```python
from build123d import *

# Parameters (mm, degrees)
SZKIC1_R                    = 3
DODANIE_WYCI_GNI_CIE1_DEPTH = 30
DODANIE_WYCI_GNI_CIE2_DEPTH = 4
SFAZOWANIE1_SIZE            = 1


with BuildPart() as part:
    # Szkic1 → Dodanie-wyciągnięcie1 (new body)
    with BuildSketch(Plane(origin=(0, 0, 0), x_dir=(1, 0, 0), z_dir=(0, 1, 0))):
        with Locations(Location((0, 0, 0), (0, 0, 270))):
            Circle(SZKIC1_R)
    extrude(amount=-DODANIE_WYCI_GNI_CIE1_DEPTH)

    # Szkic2 → Dodanie-wyciągnięcie2 (add)
    with BuildSketch(Plane(origin=(0, 0, 0), x_dir=(1, 0, 0), z_dir=(0, 1, 0))):
        Polygon((5.773502692, 0), (2.886751346, 5), (-2.886751346, 5), (-5.773502692, 0), (-2.886751346, -5), (2.886751346, -5), align=None)
    extrude(amount=DODANIE_WYCI_GNI_CIE2_DEPTH)

    # Szkic4 → Wycięcie-obrót1 (revolve, cut)
    with BuildSketch(Plane.XY):
        Polygon((5.773502692, 3.226497308), (5, 4), (5.773502692, 4), align=None)
    revolve(axis=Axis((0, 4, 0), (0, -1, 0)), mode=Mode.SUBTRACT)

    # Sfazowanie1
    sfazowanie1_edges = [part.edges().sort_by_distance(p)[0] for p in [
        (0, -30, -3),
    ]]
    chamfer(sfazowanie1_edges, length=SFAZOWANIE1_SIZE)


solid = part.part
```
Model file for the job. Use its own axes, mm. A direction names the side the tool comes from. Coordinates: 2 decimals unless noted, no trailing zeros. Loops run counter-clockwise (first coordinate to the right, second up) from the corner with the lowest first, then second, coordinate; pieces in that order, holes last. Notation, with made-up numbers: (6, -38.5) -> (21, -38.5) arc R27 ccw to (21, -15.5) -> close; hole circle Ø3 at (-6.75, 64.25). An arc over 180 degrees is marked (long way). Answer as a JSON object with one key per item and string values.
Q1. Cut at B-B (y = -14). List the corners of the cut face in (x, z).
Report:
{"outline": "circle Ø6 at (0, 0)"}
Q2. 3-axis set-ups, long thin cutter, end or side, ignore diameter. For faces 1 (the conical face through (2.6, 3.82, 4.48)), 2 (the flat face through (2.5, 0, -2.3)): which of +Z, -Z, +X, -X, +Y, -Y reach the whole face in a straight line?
Report:
{"face 1": "+Z, +X, +Y", "face 2": "-Y"}
Q3. Probe probe 1 along Y at (x, z) = (3, -1.25); probe 2 along X at (y, z) = (-4, -2.75); probe 3 along X at (y, z) = (-24.5, 1). List the from-to ranges inside material, lowest first.
Report:
{"probe 1": "y = 0 to 4", "probe 2": "x = -1.2 to 1.2", "probe 3": "x = -2.83 to 2.83"}
Q4. Flat gauge pins, fed straight in: P1, Ø1.5, axis at x = 2, y = -11, coming from the -Z side; P2, Ø4, axis at x = -2.5, y = -21.5, coming from the -Z side; P3, Ø2, axis at x = -3.5, z = -3, coming from the -Y side. Where does each tip first touch, or does it go through?
Report:
{"P1": "stops at z = -2.73", "P2": "stops at z = -2.96", "P3": "stops at y = 0"}
Q5. Cut at A-A (y = 2). List the corners of the cut face in (x, z), and give its area (3 significant figures).
Report:
{"outline": "(-5.77, 0) -> (-2.89, -5) -> (2.89, -5) -> (5.77, 0) -> (2.89, 5) -> (-2.89, 5) -> close", "area": "86.6 mm2"}
